Design review of the part built by this model. Coordinates are the model's own, in mm. Coordinates: 2 decimals unless noted, no trailing zeros. Loops run counter-clockwise (first coordinate to the right, second up) from the corner with the lowest first, then second, coordinate; pieces in that order, holes last. Notation, with made-up numbers: (78, -9) - (89, -9) arc R21 cw to (89, 10) - close; hole circle Ø3 at (89, 35.5). An arc over 180 degrees is marked (long way). Answer in a Markdown table with one row per item. Add a question column.
(1) We need section C-C, the plane x = -12. Write out the cut boundary in (y, z).
(2) To check wall thickness, follow L1, parallel to Y at x = -12, z = 6.75; L2, parallel to X at y = 10.5, z = 5.5; L3, parallel to X at y = 13, z = 5.25. State the ranges of each line that lie inside material, in increasing order. Write a range as [from, to].
(3) The part is to be moulded in two halves that separate along X. For faces 1 (the face through (13.2, 9.193, 5.577)), 2 (the face through (-11.4, 8.8, 11)), 3 (the face through (-17.3, 0.6, 0.7)), say which applies: released by +X, released by -X, zero draft, split by the parting line, or undercut.
(4) We need section B-B, the plane z = 8. Write out the cut boundary in (x, y), plus the area to 3 significant figures.
(5) We need section A-A, the plane y = 11.5. Write out the cut boundary in (x, z).
(6) Clearance check with a flat-ended pin moving along its axis: pin 1 (8.5 mm diameter, centred on x = -12, y = 11.5, fed in from -Z). State where the tip first meets the part, or that it passes through.
(7) We need section D-D, the plane z = 2. Write out the cut boundary in (x, y), plus the area to 3 significant figures.
from build123d import *

# Parameters (mm, degrees)
BOSS_EXTRUDE1_DEPTH = 23
CUT_EXTRUDE1_REACH  = 13
SKETCH2_R           = 2.6
CHAMFER1_SIZE       = 1


with BuildPart() as part:
    # Sketch1 → Boss-Extrude1 (new body)
    with BuildSketch(Plane(origin=(0, 0, 0), x_dir=(1, 0, 0), z_dir=(0, 1, 0))):
        with BuildLine():
            Line((-18, 0), (18, 0))
            Line((18, 0), (18, -11))
            Line((18, -11), (4.95, -11))
            ThreePointArc((4.95, -11), (0, -6.95), (-4.95, -11))
            Line((-4.95, -11), (-18, -11))
            Line((-18, -11), (-18, 0))
        make_face()
    extrude(amount=BOSS_EXTRUDE1_DEPTH)

    # Sketch2 → Cut-Extrude1 (cut, up to next)
    with BuildSketch(Plane.XY.offset(11), mode=Mode.PRIVATE) as cut_extrude1_sk1:
        with Locations((-12, 11.5)):
            Circle(SKETCH2_R)
    cut_extrude1_tool1 = extrude(cut_extrude1_sk1.sketch, amount=-CUT_EXTRUDE1_REACH, mode=Mode.PRIVATE) & part.part
    add(cut_extrude1_tool1.solids().sort_by_distance((-12, 11.5, 11))[0], mode=Mode.SUBTRACT)
    # Sketch2 → Cut-Extrude1 (cut, up to next)
    with BuildSketch(Plane.XY.offset(11), mode=Mode.PRIVATE) as cut_extrude1_sk2:
        with Locations((12, 11.5)):
            Circle(SKETCH2_R)
    cut_extrude1_tool2 = extrude(cut_extrude1_sk2.sketch, amount=-CUT_EXTRUDE1_REACH, mode=Mode.PRIVATE) & part.part
    add(cut_extrude1_tool2.solids().sort_by_distance((12, 11.5, 11))[0], mode=Mode.SUBTRACT)

    # Chamfer1
    chamfer1_edges = [part.edges().sort_by_distance(p)[0] for p in [
        (-18, 11.5, 0),
        (18, 11.5, 0),
        (18, 23, 5.5),
        (0, 23, 0),
        (-18, 23, 5.5),
        (0, 0, 0),
        (18, 0, 5.5),
        (-18, 0, 5.5),
    ]]
    chamfer(chamfer1_edges, length=CHAMFER1_SIZE)


solid = part.part
Responses:
| question | item | result |
|---|---|---|
| 1 | outline | (0, 1) - (1, 0) - (8.9, 0) - (8.9, 11) - (0, 11) - close; (14.1, 0) - (22, 0) - (23, 1) - (23, 11) - (14.1, 11) - close |
| 2 | L1 | y = [0, 8.9], [14.1, 23] |
| 2 | L2 | x = [-18, -14.4], [-9.6, 9.6], [14.4, 18] |
| 2 | L3 | x = [-18, -14.12], [-9.88, 9.88], [14.12, 18] |
| 3 | face 1 | undercut |
| 3 | face 2 | zero draft |
| 3 | face 3 | released by -X |
| 4 | outline | (-18, 1) - (-17, 0) - (-3.08, 0) - (-3.08, 23) - (-17, 23) - (-18, 22) - close; (3.08, 0) - (17, 0) - (18, 1) - (18, 22) - (17, 23) - (3.08, 23) - close; hole circle Ø5.2 at (-12, 11.5); hole circle Ø5.2 at (12, 11.5) |
| 4 | area | 642 mm2 |
| 5 | outline | (-18, 1) - (-17, 0) - (-14.6, 0) - (-14.6, 11) - (-18, 11) - close; (-9.4, 0) - (9.4, 0) - (9.4, 11) - (4.95, 11) arc R5.05 cw to (-4.95, 11) - (-9.4, 11) - close; (14.6, 0) - (17, 0) - (18, 1) - (18, 11) - (14.6, 11) - close |
| 6 | pin 1 | stops at z = 0 |
| 7 | outline | (-18, 1) - (-17, 0) - (17, 0) - (18, 1) - (18, 22) - (17, 23) - (-17, 23) - (-18, 22) - close; hole circle Ø5.2 at (-12, 11.5); hole circle Ø5.2 at (12, 11.5) |
| 7 | area | 784 mm2 |
